Check sheet for the modelled part. Datum: model origin and axes. Units: mm. A direction names the side the tool comes from. Round coordinates to 2 decimals unless told otherwise and drop trailing zeros. Write each loop counter-clockwise with the first axis right and the second up, starting at its lowest first coordinate (ties: lowest second). Pieces come first, ordered by that corner, then holes. Notation, with made-up numbers: M 32.25,-4.75 L 47.25,-4.75 A9 ccw 47.25,5.25 Z; hole C 48,79 d9. An arc over 180 degrees is marked long. One line per item, written item: value.
from build123d import *

# Parameters (mm, degrees)
AUFSATZ_LINEAR_AUSTRAGEN2_DEPTH = 2


with BuildPart() as part:
    # Skizze2 → Aufsatz-Linear austragen2 (new body)
    with BuildSketch(Plane(origin=(0, 0, 0), x_dir=(1, 0, 0), z_dir=(0, 1, 0))):
        with BuildLine():
            Line((-44, 50), (-28, 50))
            Line((-28, 50), (-16.61985221, 33))
            ThreePointArc((-16.61985221, 33), (0, 24.125669082), (16.61985221, 33))
            Line((16.61985221, 33), (28, 50))
            Line((28, 50), (44, 50))
            ThreePointArc((44, 50), (47.535533906, 48.535533906), (49, 45))
            Line((49, 45), (49, -49))
            Line((49, -49), (-49, -49))
            Line((-49, -49), (-49, 45))
            ThreePointArc((-49, 45), (-47.535533906, 48.535533906), (-44, 50))
        make_face()
    extrude(amount=AUFSATZ_LINEAR_AUSTRAGEN2_DEPTH)


solid = part.part
Q1. Sectioned sample at C-C on x = 9. Enter the section's corners in (y, z).
Completed:
outline: M 0,-26.27 L 2,-26.27 L 2,49 L 0,49 Z
Q2. Access from +Z, -Z, +X, -X, +Y, -Y to the whole of each face (thin tool, end or side, straight path). Record for faces 5 (the flat face through (1, 2, -1)), 6 (the flat face through (-22.39, 0.99, -41.62)).
Completed:
face 5: +Z, -Z, +X, -X, +Y
face 6: -Z, +Y, -Y
Q3. Sectioned sample at B-B on y = 0.9. Enter the section's corners in (x, z).
Completed:
outline: M -49,-45 A5 ccw -44,-50 L -28,-50 L -16.62,-33 A20 cw 16.62,-33 L 28,-50 L 44,-50 A5 ccw 49,-45 L 49,49 L -49,49 Z
Q4. Scan lines: line 1 (X direction, y = 1.5, z = -28); line 2 (X direction, y = 0.1, z = -46); line 3 (Z direction, x = 26, y = 0.65). Record each from-to range of solid material in increasing order. Write a range as [from, to].
Completed:
line 1: [-49, -11.83], [11.83, 49]
line 2: [-48.9, -25.32], [25.32, 48.9]
line 3: [-47.01, 49]
Q5. Draft check along X on faces 1 (the cylindrical face through (47, 1, -49)), 2 (the cylindrical face through (-0.275, 0.986, -24.128)), 3 (the cylindrical face through (-48, 1, -48)), 4 (the flat face through (1, 0, -1)). Enter one of: pulls with the +X half, pulls with the -X half, needs draft (parallel to the pull), parting line crosses it, or undercut.
Completed:
face 1: pulls with the +X half
face 2: undercut
face 3: pulls with the -X half
face 4: needs draft
Q6. Sectioned sample at A-A on z = -36.5. Enter the section's corners in (x, y), and give its area (3 significant figures).
Completed:
outline: M -49,0 L -18.96,0 L -18.96,2 L -49,2 Z; M 18.96,0 L 49,0 L 49,2 L 18.96,2 Z
area: 120 mm^2
Q7. Depth check by flat-ended pin: P1, Ø3, axis at x = -16, z = -26, coming from the -Y side. Enter the tip coordinate at first touch or a pass-through.
Completed:
P1: y = 0
